from build123d import *

# Parameters (mm, degrees)
SKETCH_1_W          = 64
SKETCH_1_H          = 64
EXTRUDE_1_DEPTH     = 11
SKETCH_2_R          = 17.6
SKETCH_2_R_2        = 2.1
CUT_EXTRUDE_1_DEPTH = 11
FILLET_1_R          = 10


with BuildPart() as part:
    # 草图1 → 凸台-拉伸1 (new body)
    with BuildSketch(Plane(origin=(0, 0, 0), x_dir=(1, 0, 0), z_dir=(0, 1, 0))):
        Rectangle(SKETCH_1_W, SKETCH_1_H)
    extrude(amount=EXTRUDE_1_DEPTH)

    # 草图2 → 切除-拉伸1 (cut)
    with BuildSketch(Plane(origin=(0, 11, 0), x_dir=(1, 0, 0), z_dir=(0, 1, 0))):
        with Locations(Location((0, 0, 0), (0, 0, 270))):
            Circle(SKETCH_2_R)
        with Locations(Location((24.04163056, 24.04163056, 0), (0, 0, 270))):
            Circle(SKETCH_2_R_2)
        with Locations(Location((24.04163056, -24.04163056, 0), (0, 0, 270))):
            Circle(SKETCH_2_R_2)
        with Locations(Location((-24.04163056, -24.04163056, 0), (0, 0, 270))):
            Circle(SKETCH_2_R_2)
        with Locations(Location((-24.04163056, 24.04163056, 0), (0, 0, 270))):
            Circle(SKETCH_2_R_2)
    extrude(amount=-CUT_EXTRUDE_1_DEPTH, mode=Mode.SUBTRACT)

    # 圆角1
    fillet_1_edges = [part.edges().sort_by_distance(p)[0] for p in [
        (32, 5.5, 32),
        (-32, 5.5, 32),
        (-32, 5.5, -32),
        (32, 5.5, -32),
    ]]
    fillet(fillet_1_edges, radius=FILLET_1_R)


solid = part.part
Geometry: final body of the model. Coordinates: model frame, mm. Give positions to 0.01 mm unless a question says otherwise; leave off trailing zeros. Loops run counter-clockwise (first coordinate to the right, second up) from the corner with the lowest first, then second, coordinate; pieces in that order, holes last. Notation, with made-up numbers: (26.5, 40.5) - (82.5, 40.5) arc R29 ccw to (82.5, 69.5) - close; hole circle Ø6 at (1, 1.5). An arc over 180 degrees is marked (long way). Answer as CSV lines item,"result". Start each with the question number.
1. Section C-C, the plane x = -23. Return loops of the section in (y, z), plus the area to 3 significant figures.
2. Section A-A, the plane z = 0. Return loops of the section in (x, y).
3. Section D-D, the plane y = 3. Return loops of the section in (x, z), plus the area to 3 significant figures.
4. Draft query along X for faces 1 (the face through (-29.15, 5.58, 28.99)), 2 (the face through (32, 5, 0)), 3 (the face through (-21.96, 5.58, 23.77)). Return one class per face: released by +X, released by -X, zero draft, split by the parting line, or undercut.
5. Section B-B, the plane x = 0. Return loops of the section in (y, z), plus the area to 3 significant figures.
6. Pin query (flat end, axial travel): P1, Ø5, axis at x = 24.04, z = 24.04, coming from the +Y side. Return the tip coordinate at first contact, or that it passes through.
7. Ray query, L1, parallel to X at y = 6, z = 0; L2, parallel to Z at x = 0.5, y = 9; L3, parallel to Z at x = -25.5, y = 6.75. Return the intervals inside material, ascending.
Answers:
1,outline,"(0, -31.95) - (11, -31.95) - (11, -25.87) - (0, -25.87) - close; (0, -22.22) - (11, -22.22) - (11, 22.22) - (0, 22.22) - close; (0, 25.87) - (11, 25.87) - (11, 31.95) - (0, 31.95) - close"
1,area,"623 mm2"
2,outline,"(-32, 0) - (-17.6, 0) - (-17.6, 11) - (-32, 11) - close; (17.6, 0) - (32, 0) - (32, 11) - (17.6, 11) - close"
3,outline,"(-32, -22) arc R10 ccw to (-22, -32) - (22, -32) arc R10 ccw to (32, -22) - (32, 22) arc R10 ccw to (22, 32) - (-22, 32) arc R10 ccw to (-32, 22) - close; hole circle Ø4.2 at (-24.04, -24.04); hole circle Ø4.2 at (-24.04, 24.04); hole circle Ø35.2 at (0, 0); hole circle Ø4.2 at (24.04, -24.04); hole circle Ø4.2 at (24.04, 24.04)"
3,area,"2,980 mm2"
4,face 1,"released by -X"
4,face 2,"released by +X"
4,face 3,"undercut"
5,outline,"(0, -32) - (11, -32) - (11, -17.6) - (0, -17.6) - close; (0, 17.6) - (11, 17.6) - (11, 32) - (0, 32) - close"
5,area,"317 mm2"
6,P1,"stops at y = 11"
7,L1,"x = -32 to -17.6, 17.6 to 32"
7,L2,"z = -32 to -17.59, 17.59 to 32"
7,L3,"z = -31.37 to -25.55, -22.53 to 22.53, 25.55 to 31.37"
